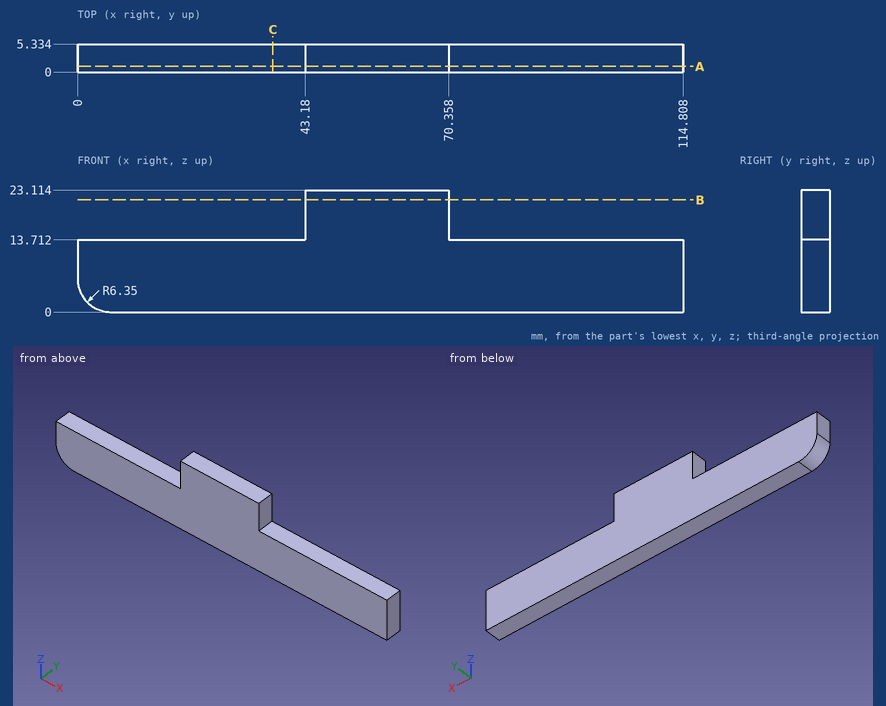
Study the drawing (mm; zero at the part's minimum x, y, z) and answer. Give positions to 0.01 mm unless a question says otherwise; leave off trailing zeros. Write each loop counter-clockwise with the first axis right and the second up, starting at its lowest first coordinate (ties: lowest second). Pieces come first, ordered by that corner, then holes.
(1) The part is cut by section A-A on y = 1.1. Write down the section's boundary in (x, z), plus the area to 3 significant figures.
Final values:
outline: (0, 6.35) arc R6.35 ccw to (6.35, 0) - (114.81, 0) - (114.81, 13.71) - (70.36, 13.71) - (70.36, 23.11) - (43.18, 23.11) - (43.18, 13.71) - (0, 13.71) - close
area: 1,820 mm2
(2) Straight lines are drawn through the part: line 1 (Z direction, x = 104, y = 0.7); line 2 (X direction, y = 3.6, z = 18.5); line 3 (X direction, y = 2, z = 2) (1 decimal). For each, find the intervals that lie inside material, in ascending order.
Final values:
line 1: z = 0 to 13.71
line 2: x = 43.18 to 70.36
line 3: x = 1.7 to 114.8
(3) Flat-ended cylindrical pins translate along their axes: pin 1 Ø1 at (y, z) = (2.5, 15) entering from +X; pin 2 Ø3 at (x, y) = (89.5, 1.5) entering from +Z; pin 3 Ø1.6 at (y, z) = (2.5, 20.5) entering from -X. Find the tip coordinate at first contact, or state that the pin passes through.
Final values:
pin 1: stops at x = 70.36
pin 2: stops at z = 13.71
pin 3: stops at x = 43.18
(4) The part is cut by section B-B on z = 21.25. Write down the section's boundary in (x, y), plus the area to 3 significant figures.
Final values:
outline: (43.18, 0) - (70.36, 0) - (70.36, 5.33) - (43.18, 5.33) - close
area: 145 mm2
(5) The part is cut by section C-C on x = 37. Write down the section's boundary in (y, z).
Final values:
outline: (0, 0) - (5.33, 0) - (5.33, 13.71) - (0, 13.71) - close
